```python
from build123d import *

# Parameters (mm, degrees)
F0_W      = 33.02
F0_H      = 25.4
F1_DEPTH  = 10.795
F2_W      = 22.86
F2_H      = 19.05
F3_DEPTH  = 48.26
F4_W      = 33.02
F4_H      = 15.24
F5_DEPTH  = 12.7
F6_W      = 33.02
F6_H      = 15.24
F7_DEPTH  = 48.26
F8_W      = 12.7
F8_H      = 12.7
F9_DEPTH  = 2.54
F10_W     = 7.112
F10_H     = 69.85
F11_DEPTH = 12.7
F13_R     = 6.033573
F14_DEPTH = 6.35
F12_R     = 9.525
F15_DEPTH = 3.81
F16_R     = 9.525
F17_DEPTH = 3.81
F18_R     = 9.525
F19_DEPTH = 3.81
F20_R     = 9.525
F21_DEPTH = 3.81
F22_R     = 9.525
F23_DEPTH = 3.81
F24_R     = 9.525
F25_DEPTH = 3.81
F26_R     = 6.066137
F27_DEPTH = 6.35
F28_W     = 73.66
F28_H     = 8.89
F29_DEPTH = 1.27
F30_W     = 73.66
F30_H     = 8.89
F31_DEPTH = 1.27
F32_W     = 73.66
F32_H     = 2.54
F33_DEPTH = 1.27
F34_W     = 73.66
F34_H     = 2.54
F35_DEPTH = 1.27
F36_W     = 4.064
F36_H     = 2.54
F37_DEPTH = 1.27


with BuildPart() as f1:
    # F0 (on Front) → F1 (new body, symmetric)
    with BuildSketch(Plane.XZ):
        Rectangle(F0_W, F0_H)
    extrude(amount=F1_DEPTH, both=True)

    # F2 (on face) → F3 (join)
    with BuildSketch(Plane.XZ.offset(10.795)):
        with Locations((0, -3.175)):
            Rectangle(F2_W, F2_H)
    extrude(amount=F3_DEPTH)

    # F4 (on Front) → F5 (join, symmetric)
    with BuildSketch(Plane.XZ):
        with Locations((0, -20.32)):
            Rectangle(F4_W, F4_H)
    extrude(amount=F5_DEPTH, both=True)

    # F6 (on face) → F7 (join)
    with BuildSketch(Plane.XZ.offset(12.7)):
        with Locations((0, -20.32)):
            Rectangle(F6_W, F6_H)
    extrude(amount=F7_DEPTH)

    # F8 (on face) → F9 (join)
    with BuildSketch(Plane.XZ.offset(59.055)):
        with Locations((0, -6.35)):
            Rectangle(F8_W, F8_H)
    extrude(amount=F9_DEPTH)

    # F10 (on face) → F11 (cut)
    with BuildSketch(Plane(origin=(0, 0, -27.94), x_dir=(1, 0, 0), z_dir=(0, 0, -1))):
        with Locations((-11.934741, 24.13)):
            Rectangle(F10_W, F10_H)
        with Locations((12.118584, 24.13)):
            Rectangle(F10_W, F10_H)
    extrude(amount=-F11_DEPTH, mode=Mode.SUBTRACT)

    # F13 (on face) → F14 (join)
    with BuildSketch(Plane.XZ.offset(60.96)):
        with Locations((0, -20.813061)):
            Circle(F13_R)
    extrude(amount=F14_DEPTH)

    # F12 (on face) → F15 (join)
    with BuildSketch(Plane(origin=(-8.378741, 0, 0), x_dir=(0, -1, 0), z_dir=(-1, 0, 0))):
        with Locations((24.13, -27.94)):
            Circle(F12_R)
    extrude(amount=F15_DEPTH)

    # F16 (on face) → F17 (join)
    with BuildSketch(Plane(origin=(-8.378741, 0, 0), x_dir=(0, -1, 0), z_dir=(-1, 0, 0))):
        with Locations((46.355, -27.94)):
            Circle(F16_R)
    extrude(amount=F17_DEPTH)

    # F18 (on face) → F19 (join)
    with BuildSketch(Plane(origin=(-8.378741, 0, 0), x_dir=(0, -1, 0), z_dir=(-1, 0, 0))):
        with Locations((1.905, -27.94)):
            Circle(F18_R)
    extrude(amount=F19_DEPTH)

    # F20 (on face) → F21 (join)
    with BuildSketch(Plane.YZ.offset(8.562584)):
        with Locations((-24.13, -27.94)):
            Circle(F20_R)
    extrude(amount=F21_DEPTH)

    # F22 (on face) → F23 (join)
    with BuildSketch(Plane.YZ.offset(8.562584)):
        with Locations((-1.905, -27.94)):
            Circle(F22_R)
    extrude(amount=F23_DEPTH)

    # F24 (on face) → F25 (join)
    with BuildSketch(Plane.YZ.offset(8.562584)):
        with Locations((-46.355, -27.94)):
            Circle(F24_R)
    extrude(amount=F25_DEPTH)

    # F26 (on face) → F27 (join)
    with BuildSketch(Plane(origin=(0, 12.7, 0), x_dir=(-1, 0, 0), z_dir=(0, 1, 0))):
        with Locations((0.010551, -20.824138)):
            Circle(F26_R)
    extrude(amount=F27_DEPTH)

    # F28 (on face) → F29 (join)
    with BuildSketch(Plane.YZ.offset(16.51)):
        with Locations((-24.13, -23.495)):
            Rectangle(F28_W, F28_H)
    extrude(amount=F29_DEPTH)

    # F30 (on face) → F31 (join)
    with BuildSketch(Plane(origin=(-16.51, 0, 0), x_dir=(0, -1, 0), z_dir=(-1, 0, 0))):
        with Locations((24.13, -23.495)):
            Rectangle(F30_W, F30_H)
    extrude(amount=F31_DEPTH)

    # F32 (on face) → F33 (join)
    with BuildSketch(Plane.YZ.offset(17.78)):
        with Locations((-24.13, -26.67)):
            Rectangle(F32_W, F32_H)
    extrude(amount=F33_DEPTH)

    # F34 (on face) → F35 (join)
    with BuildSketch(Plane(origin=(-17.78, 0, 0), x_dir=(0, -1, 0), z_dir=(-1, 0, 0))):
        with Locations((24.13, -26.67)):
            Rectangle(F34_W, F34_H)
    extrude(amount=F35_DEPTH)

    # F36 (on face) → F37 (cut)
    with BuildSketch(Plane(origin=(0, 10.795, 0), x_dir=(-1, 0, 0), z_dir=(0, 1, 0))):
        with Locations((-0.015461, -11.43)):
            Rectangle(F36_W, F36_H)
    extrude(amount=-F37_DEPTH, mode=Mode.SUBTRACT)


solid = f1.part
```
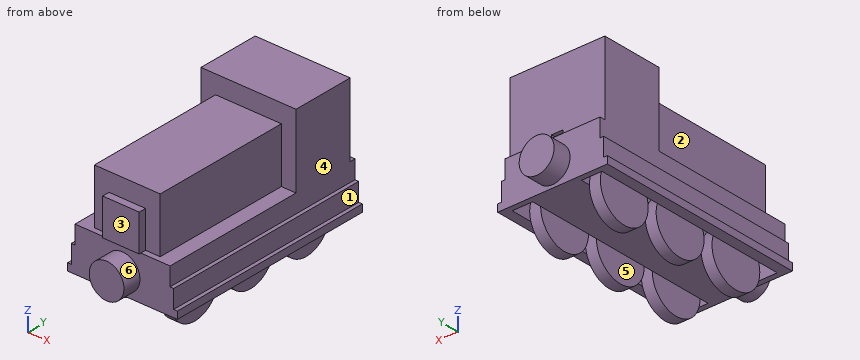
The listing builds one solid part. Answer for the finished solid, in the listing's coordinates (mm). Face numbers are marked on the shaded views. A direction names the side the tool comes from. Coordinates: 2 decimals unless noted, no trailing zeros. Order: outer loops, then holes, each group sorted by start corner. A loop starts at its lowest first (then second) coordinate and runs counter-clockwise, first axis right, second up. Notation, with made-up numbers: M 54.25,19 L 76.25,19 A20 cw 76.25,47 Z; hole C 75.5,9.25 d11. An arc over 180 degrees is marked long. Answer as a JSON object with one key per item and string values. Group by question number.
1. Section D-D on z = -17 is taken. Write down the section's boundary in (x, y) (3 decimals), then the cut area to 3 significant figures.
2. Section B-B on z = -2 is taken. Write down the section's boundary in (x, y) (3 decimals), then the cut area to 3 significant figures.
3. Section A-A on x = -7.5 is taken. Write down the section's boundary in (y, z) (3 decimals).
4. A tool of negligible diameter and unlimited length cuts with its end or side. For the marked faces 1, 2 and 3, from which of +Z, -Z, +X, -X, +Y, -Y can it reach the whole face along a straight path? Write none if from no direction.
5. Straight lines are drawn through the part: line 1 (X direction, y = -22.5, z = -17.5); line 2 (Y direction, x = -10, z = -33.5); line 3 (Z direction, x = 14, y = -30.5). For each, find the intervals that lie inside material, in ascending order.
6. Determine the mould class of the marked faces 4, 5 and 6 for opening direction X: released by +X, released by -X, zero draft, split by the parting line, or undercut.
7. Flat-ended cylindrical pins translate along their axes: P1, Ø1.4, axis at y = 10, z = -12, coming from the -X side; P2, Ø2, axis at x = 12.5, y = -23, coming from the -Z side; P3, Ø3, axis at y = -60, z = -9, coming from the +X side; P4, Ø5, axis at x = 10, y = -36.5, coming from the +Z side. Find the tip coordinate at first contact, or state that the pin passes through.
Values follow:
{
 "1": {"outline": "M -16.51,-60.96 L -4.676,-60.96 L -4.676,-67.31 L 4.676,-67.31 L 4.676,-60.96 L 16.51,-60.96 L 16.51,12.7 L 4.698,12.7 L 4.698,19.05 L -4.719,19.05 L -4.719,12.7 L -16.51,12.7 Z; hole M -15.491,-59.055 L -8.379,-59.055 L -8.379,10.795 L -15.491,10.795 Z; hole M 8.563,-59.055 L 15.675,-59.055 L 15.675,10.795 L 8.563,10.795 Z", "area": "1,560 mm2"},
 "2": {"outline": "M -16.51,-10.795 L -11.43,-10.795 L -11.43,-59.055 L -6.35,-59.055 L -6.35,-61.595 L 6.35,-61.595 L 6.35,-59.055 L 11.43,-59.055 L 11.43,-10.795 L 16.51,-10.795 L 16.51,10.795 L -16.51,10.795 Z", "area": "1,850 mm2"},
 "3": {"outline": "M -60.96,-27.94 L 12.7,-27.94 L 12.7,-12.7 L 10.795,-12.7 L 10.795,12.7 L -10.795,12.7 L -10.795,6.35 L -59.055,6.35 L -59.055,-12.7 L -60.96,-12.7 Z"},
 "4": {"face 1": "+Z, +X, +Y, -Y", "face 2": "+Z, -X, -Y", "face 3": "+Z, +X, -X, -Y"},
 "5": {"line 1": "-16.51 to -15.49, -8.38 to 8.56, 15.67 to 16.51", "line 2": "-54.09 to -38.62, -31.86 to -16.4, -9.64 to 5.83", "line 3": "-15.24 to -12.7"},
 "6": {"face 4": "released by +X", "face 5": "undercut", "face 6": "split by the parting line"},
 "7": {"P1": "x = -16.51", "P2": "z = -37.46", "P3": "x = 11.43", "P4": "z = 6.35"}
}
